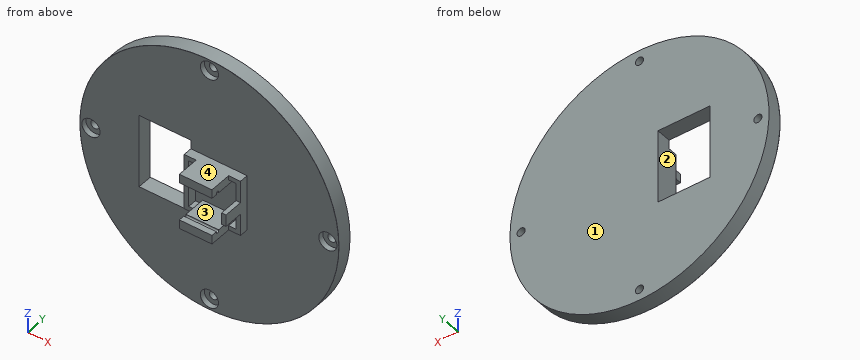
from build123d import *

# Parameters (mm, degrees)
SKETCH1_R                              = 87.5
BOSS_EXTRUDE1_DEPTH                    = 10
SKETCH2_R                              = 7.5
BOSS_EXTRUDE2_DEPTH                    = 80
CBORE_FOR_M5_HEX_HEAD_BOLT1_AT_2_COUNT = 2
CBORE_FOR_M5_HEX_HEAD_BOLT1_AT_2_PITCH = 113.13708499
CBORE_FOR_M5_HEX_HEAD_BOLT1_AT_3_COUNT = 2
CBORE_FOR_M5_HEX_HEAD_BOLT1_AT_3_PITCH = 160
CBORE_FOR_M5_HEX_HEAD_BOLT1_AT_4_COUNT = 2
CBORE_FOR_M5_HEX_HEAD_BOLT1_AT_4_PITCH = 113.13708499
SKETCH5_R                              = 87.5
CUT_EXTRUDE1_DEPTH                     = 80
FILLET1_R                              = 0.1
SKETCH10_W                             = 35
SKETCH10_H                             = 50
CUT_EXTRUDE3_DEPTH                     = 23
SKETCH12_W                             = 38
SKETCH12_H                             = 38
BOSS_EXTRUDE3_DEPTH                    = 6
SKETCH13_W                             = 22
SKETCH13_H                             = 6
BOSS_EXTRUDE4_DEPTH                    = 15
SKETCH14_W                             = 3
SKETCH14_H                             = 8
BOSS_EXTRUDE5_DEPTH                    = 13
CUT_EXTRUDE4_DEPTH                     = 93.0000001


with BuildPart() as part:
    # Sketch1 → Boss-Extrude1 (new body)
    with BuildSketch(Plane(origin=(0, 0, 0), x_dir=(1, 0, 0), z_dir=(0, 1, 0))):
        Circle(SKETCH1_R)
    extrude(amount=BOSS_EXTRUDE1_DEPTH)

    # Sketch2 → Boss-Extrude2 (add)
    with BuildSketch(Plane(origin=(0, 10, 0), x_dir=(1, 0, 0), z_dir=(0, 1, 0))):
        with Locations((0, -80)):
            Circle(SKETCH2_R)
        with Locations((-80, 0)):
            Circle(SKETCH2_R)
        with Locations((0, 80)):
            Circle(SKETCH2_R)
        with Locations((80, 0)):
            Circle(SKETCH2_R)
    extrude(amount=BOSS_EXTRUDE2_DEPTH)

    # Sketch4 → CBORE for M5 Hex Head Bolt1 (revolve, cut)
    with BuildSketch(Plane(origin=(80, 0, 0), x_dir=(0, 0, -1), z_dir=(1, 0, 0))):
        Polygon((0, 0), (0, 21.652366702), (2.75, 20), (2.75, 3.58), (6.12, 3.58), (6.12, 0.025), (6.145, 0), align=None)
    cbore_for_m5_hex_head_bolt1 = revolve(axis=Axis((80, -6.35, 0), (0, 1, 0)), mode=Mode.SUBTRACT)

    # CBORE for M5 Hex Head Bolt1 at 2: CBORE for M5 Hex Head Bolt1 ×2
    with Locations(*[Vector(-0.707106781, 0, -0.707106781) * (i * CBORE_FOR_M5_HEX_HEAD_BOLT1_AT_2_PITCH) for i in range(1, CBORE_FOR_M5_HEX_HEAD_BOLT1_AT_2_COUNT)]):
        add(cbore_for_m5_hex_head_bolt1, mode=Mode.SUBTRACT)

    # CBORE for M5 Hex Head Bolt1 at 3: CBORE for M5 Hex Head Bolt1 ×2
    with Locations(*[(-i * CBORE_FOR_M5_HEX_HEAD_BOLT1_AT_3_PITCH, 0, 0) for i in range(1, CBORE_FOR_M5_HEX_HEAD_BOLT1_AT_3_COUNT)]):
        add(cbore_for_m5_hex_head_bolt1, mode=Mode.SUBTRACT)

    # CBORE for M5 Hex Head Bolt1 at 4: CBORE for M5 Hex Head Bolt1 ×2
    with Locations(*[Vector(-0.707106781, 0, 0.707106781) * (i * CBORE_FOR_M5_HEX_HEAD_BOLT1_AT_4_PITCH) for i in range(1, CBORE_FOR_M5_HEX_HEAD_BOLT1_AT_4_COUNT)]):
        add(cbore_for_m5_hex_head_bolt1, mode=Mode.SUBTRACT)

    # Sketch5 → Cut-Extrude1 (cut)
    with BuildSketch(Plane(origin=(0, 10, 0), x_dir=(1, 0, 0), z_dir=(0, 1, 0))):
        Circle(SKETCH5_R)
    extrude(amount=CUT_EXTRUDE1_DEPTH, mode=Mode.SUBTRACT)

    # Fillet1
    fillet1_edges = [part.edges().sort_by_distance(p)[0] for p in [
        (-87.5, 0, 0),
    ]]
    fillet(fillet1_edges, radius=FILLET1_R)

    # Sketch10 → Cut-Extrude3 (cut)
    with BuildSketch(Plane(origin=(0, 10, 0), x_dir=(1, 0, 0), z_dir=(0, 1, 0))):
        with Locations((-30, 0)):
            Rectangle(SKETCH10_W, SKETCH10_H)
    extrude(amount=-CUT_EXTRUDE3_DEPTH, mode=Mode.SUBTRACT)

    # Sketch12 → Boss-Extrude3 (add)
    with BuildSketch(Plane.XZ):
        with Locations((6.5, 0)):
            Rectangle(SKETCH12_W, SKETCH12_H)
        Polygon((22.5, 16), (17.5, 16), (17.5, 13), (-4.5, 13), (-4.5, 16), (-9.5, 16), (-9.5, -16), (-4.5, -16), (-4.5, -13), (17.5, -13), (17.5, -16), (22.5, -16), align=None, mode=Mode.SUBTRACT)
    extrude(amount=BOSS_EXTRUDE3_DEPTH)

    # Sketch13 → Boss-Extrude4 (add)
    with BuildSketch(Plane.XZ.offset(6)):
        with Locations((6.5, 16)):
            Rectangle(SKETCH13_W, SKETCH13_H)
        with Locations((6.5, -16)):
            Rectangle(SKETCH13_W, SKETCH13_H)
    extrude(amount=BOSS_EXTRUDE4_DEPTH)

    # Sketch14 → Boss-Extrude5 (add)
    with BuildSketch(Plane.XZ.offset(6)):
        with Locations((24, 0)):
            Rectangle(SKETCH14_W, SKETCH14_H)
    extrude(amount=BOSS_EXTRUDE5_DEPTH)

    # Sketch15 → Cut-Extrude4 (cut, through all)
    with BuildSketch(Plane.ZY.offset(4.5)):
        with BuildLine():
            ThreePointArc((-13.500000002, -17.1), (-12.4, -16.000000001), (-13.5, -14.9))
            ThreePointArc((-13.5, -14.9), (-14.6, -15.999999999), (-13.500000002, -17.1))
        make_face()
        with BuildLine():
            ThreePointArc((13.500000002, -17.1), (14.6, -15.999999999), (13.5, -14.9))
            ThreePointArc((13.5, -14.9), (12.4, -16.000000001), (13.500000002, -17.1))
        make_face()
    extrude(amount=-CUT_EXTRUDE4_DEPTH, mode=Mode.SUBTRACT)


solid = part.part
Here's how the part is built. I have some questions about the finished solid (model axes, mm). Face numbers are marked on the shaded views. A direction names the side the tool comes from. Coordinates: 2 decimals unless noted, no trailing zeros.
Item 1: I want a section at A-A on z = 0. Count the separate pieces of the cut face and the enclosed holes in it, and give its area (3 significant figures).
Item 2: If I drill on line 1 (X direction, y = 8.5, z = 0); line 2 (Z direction, x = 11, y = -16); line 3 (Z direction, x = 10.5, y = -13), over which ranges is the centre line in solid material (lowest first)?
Item 3: On a 3-axis mill with a long thin cutter (end or side, diameter ignored), from which of +Z, -Z, +X, -X, +Y, -Y can I reach the whole of each face in a straight line? I mean the marked faces 3 and 4. Say none if no direction works.
Item 4: If we mould it in two halves opening along X, with no side actions, what happens to the marked faces 1 and 2? For each: +X half, -X half, draft (parallel to the pull), parting line (faces both ways), or undercut.
Item 5: Will these pins go through, and if not, where does the flat tip stop? pin 1 (2 mm diameter, centred on y = 3, z = 59.5, fed in from -X); pin 2 (6.5 mm diameter, centred on x = 80, z = 0, fed in from -Y); pin 3 (10 mm diameter, centred on x = -10, y = -12.5, fed in from +Z) (3 decimals); pin 4 (12 mm diameter, centred on x = -23.5, z = -33, fed in from -Y).
Findings below:
1. separate pieces: 4
1. enclosed holes: 0
1. area: 1,320 mm2
2. line 1: x = -87.5 to -82.75, -77.25 to -47.5, -12.5 to 77.25, 82.75 to 87.5
2. line 2: z = -19 to -14.6, 14.6 to 19
2. line 3: z = -19 to -13, 13 to 19
3. face 3: -Y
3. face 4: +Z, +X, -X, -Y
4. face 1: draft
4. face 2: undercut
5. pin 1: stops at x = -65.07
5. pin 2: stops at y = 3.58
5. pin 3: passes through
5. pin 4: stops at y = 0
